Source: three-view drawing plus pictorial views. Frame: mm from the lowest corner of the part. A direction names the side the tool comes from. Give positions to 0.01 mm unless a question says otherwise; leave off trailing zeros. Write each loop counter-clockwise with the first axis right and the second up, starting at its lowest first coordinate (ties: lowest second). Pieces come first, ordered by that corner, then holes. Notation, with made-up numbers: M 15.5,31.25 L 71.5,31.25 A29 ccw 71.5,67.25 Z; hole C 74.25,82 d7. An arc over 180 degrees is marked long. Return JSON: item names as keys, results as strings.
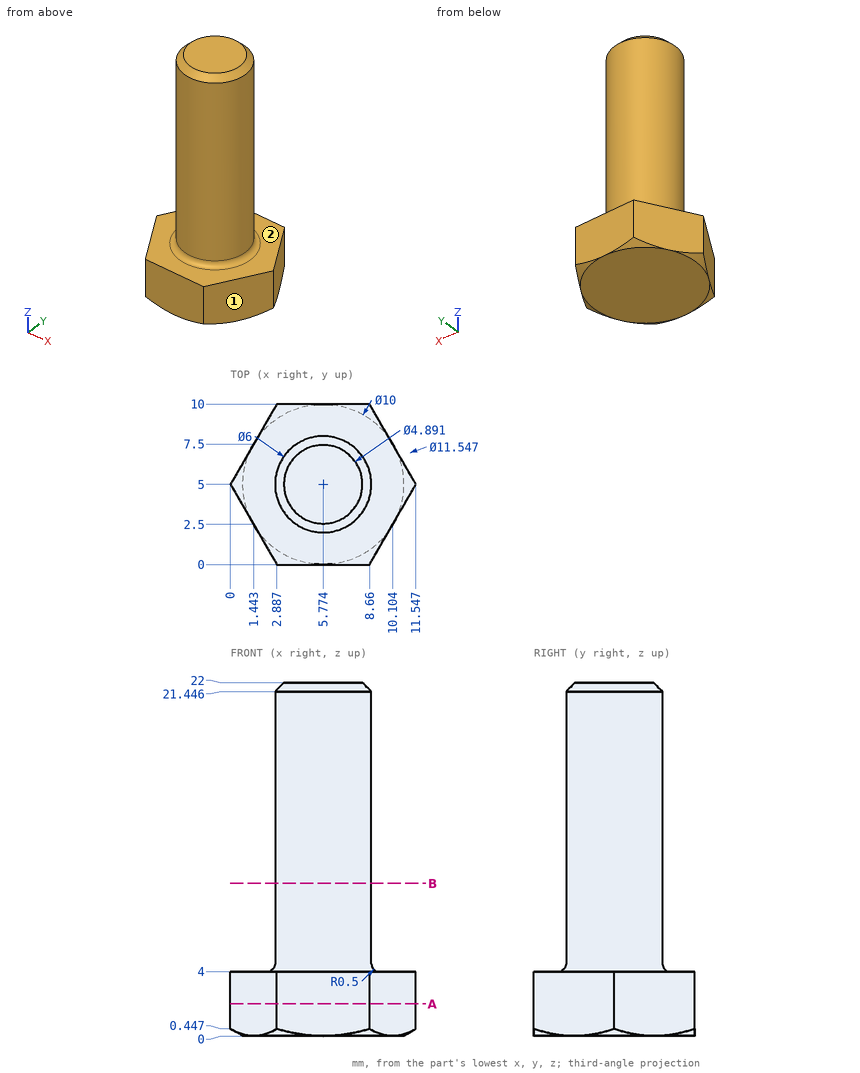
1) Set-up query: the marked faces 1 and 2. Return all of +Z, -Z, +X, -X, +Y, -Y with unobstructed straight access to the full face (end or side cutting, diameter ignored); none if empty.
Numbers:
{"face 1": "+Z, -Z, +X, -Y", "face 2": "+Z"}
2) Cut plane B-B, the plane z = 9.5. Return the cut outline in (x, y).
Numbers:
{"outline": "C 5.77,5 d6"}
3) Line query: line 1 (Z direction, x = 5.5, y = 9.5); line 2 (X direction, y = 6.5, z = 3.5) (1 decimal); line 3 (X direction, y = 4, z = 5.5) (1 decimal). Output: solid intervals per line, ascending. Write a range as [from, to].
Numbers:
{"line 1": "z = [0, 4]", "line 2": "x = [0.9, 10.7]", "line 3": "x = [2.9, 8.6]"}
4) Contact query for a flat-ended pin moving along its axis: pin 1 Ø2 at (y, z) = (7.5, 12) entering from -X (1 decimal). Output: stop coordinate, or through.
Numbers:
{"pin 1": "stops at x = 3.2"}
5) Cut plane A-A, the plane z = 2. Return the cut outline in (x, y).
Numbers:
{"outline": "M 0,5 L 2.89,0 L 8.66,0 L 11.55,5 L 8.66,10 L 2.89,10 Z"}
